from build123d import *

# Parameters (mm, degrees)
BODYSKE_R  = 0.85
BODY_DEPTH = 1


with BuildPart() as part:
    # BodySke → Body (new body)
    with BuildSketch(Plane.XY):
        with BuildLine():
            Line((0.158839779, -5.747805662), (0.25, -9.046546302))
            ThreePointArc((0.25, -9.046546302), (1.577173754, -8.9115107), (2.870077767, -8.582840649))
            ThreePointArc((2.870077767, -8.582840649), (3.210901949, -8.348665738), (3.375809664, -7.969450157))
            Line((3.375809664, -7.969450157), (3.567937091, -6.510097462))
            ThreePointArc((3.567937091, -6.510097462), (3.852773959, -5.652106923), (4.435031511, -4.960546405))
            ThreePointArc((4.435031511, -4.960546405), (0, 7.55), (-4.435031511, -4.960546405))
            ThreePointArc((-4.435031511, -4.960546405), (-3.852773959, -5.652106923), (-3.567937091, -6.510097462))
            Line((-3.567937091, -6.510097462), (-3.375809664, -7.969450157))
            ThreePointArc((-3.375809664, -7.969450157), (-3.210901949, -8.348665738), (-2.870077767, -8.582840649))
            ThreePointArc((-2.870077767, -8.582840649), (-1.577173754, -8.9115107), (-0.25, -9.046546302))
            Line((-0.25, -9.046546302), (-0.158839779, -5.747805662))
            ThreePointArc((-0.158839779, -5.747805662), (0, 5.75), (0.158839779, -5.747805662))
        make_face()
        with Locations((1.35, -7.402913278)):
            Circle(BODYSKE_R, mode=Mode.SUBTRACT)
        with Locations((-1.35, -7.402913278)):
            Circle(BODYSKE_R, mode=Mode.SUBTRACT)
    extrude(amount=-BODY_DEPTH)


solid = part.part
Source: CAD feature listing. Evaluate the final solid. Frame: model axes, mm. Give positions to 0.01 mm unless a question says otherwise; leave off trailing zeros. Write each loop counter-clockwise with the first axis right and the second up, starting at its lowest first coordinate (ties: lowest second). Pieces come first, ordered by that corner, then holes. Notation, with made-up numbers: M 55,-28 L 94,-28 A22 cw 94,1 Z; hole C 21.5,0.25 d4. An arc over 180 degrees is marked long. Answer as a JSON object with one key per item and string values.
Q1. Cut plane C-C, the plane z = -0.35. Return the cut outline in (x, y).
Geometry check:
{"outline": "M -4.44,-4.96 A2.4 cw -3.57,-6.51 L -3.38,-7.97 A0.75 ccw -2.87,-8.58 A9.05 ccw -0.25,-9.05 L -0.16,-5.75 A5.75 cw long 0.16,-5.75 L 0.25,-9.05 A9.05 ccw 2.87,-8.58 A0.75 ccw 3.38,-7.97 L 3.57,-6.51 A2.4 cw 4.44,-4.96 A7.04 ccw long Z; hole C -1.35,-7.4 d1.7; hole C 1.35,-7.4 d1.7"}
Q2. Ray query, line 1 along Y through (x, z) = (1.35, -0.4); line 2 along Y through (x, z) = (2, -0.9); line 3 along X through (y, z) = (-1.25, -0.6). Return the intervals inside material, ascending.
Geometry check:
{"line 1": "y = -8.95 to -8.25, -6.55 to -5.59, 5.59 to 7.42", "line 2": "y = -8.83 to -7.95, -6.86 to -5.39, 5.39 to 7.26", "line 3": "x = -6.82 to -5.61, 5.61 to 6.82"}
Q3. Cut plane B-B, the plane x = -3.75. Return the cut outline in (y, z), then the cut area to 3 significant figures.
Geometry check:
{"outline": "M -5.86,-1 L -4.36,-1 L -4.36,0 L -5.86,0 Z; M 4.36,-1 L 6.47,-1 L 6.47,0 L 4.36,0 Z", "area": "3.61 mm^2"}
Q4. Mould query, pull axis Y, two halves, no side actions, for faces 1 (the face through (-6, 1, 0)), 2 (the face through (-0.251, 5.745, -0.493)), 3 (the face through (3.47, -7.25, -0.49)). Classes: +Y half, -Y half, draft (parallel to the pull), parting line (faces both ways), or undercut.
Geometry check:
{"face 1": "draft", "face 2": "undercut", "face 3": "-Y half"}
Q5. Cut plane A-A, the plane y = 0. Return the cut outline in (x, z).
Geometry check:
{"outline": "M -7.02,-1 L -5.75,-1 L -5.75,0 L -7.02,0 Z; M 5.75,-1 L 7.02,-1 L 7.02,0 L 5.75,0 Z"}
Q6. Cut plane D-D, the plane x = 1.35. Return the cut outline in (y, z), then the cut area to 3 significant figures.
Geometry check:
{"outline": "M -8.95,-1 L -8.25,-1 L -8.25,0 L -8.95,0 Z; M -6.55,-1 L -5.59,-1 L -5.59,0 L -6.55,0 Z; M 5.59,-1 L 7.42,-1 L 7.42,0 L 5.59,0 Z", "area": "3.49 mm^2"}
